Drawing for the job (mm, zero at the part's lowest x, y, z). A direction names the side the tool comes from. Give positions to 0.01 mm unless a question says otherwise; leave off trailing zeros. Write each loop counter-clockwise with the first axis right and the second up, starting at its lowest first coordinate (ties: lowest second). Pieces come first, ordered by that corner, then holes. Notation, with made-up numbers: (63.5, 9.5) - (81.5, 9.5) arc R21 cw to (81.5, 23.5) - close; hole circle Ø9 at (19, 15.25). An arc over 180 degrees is marked (long way). Write item = value, one per line. Start each with the question number.
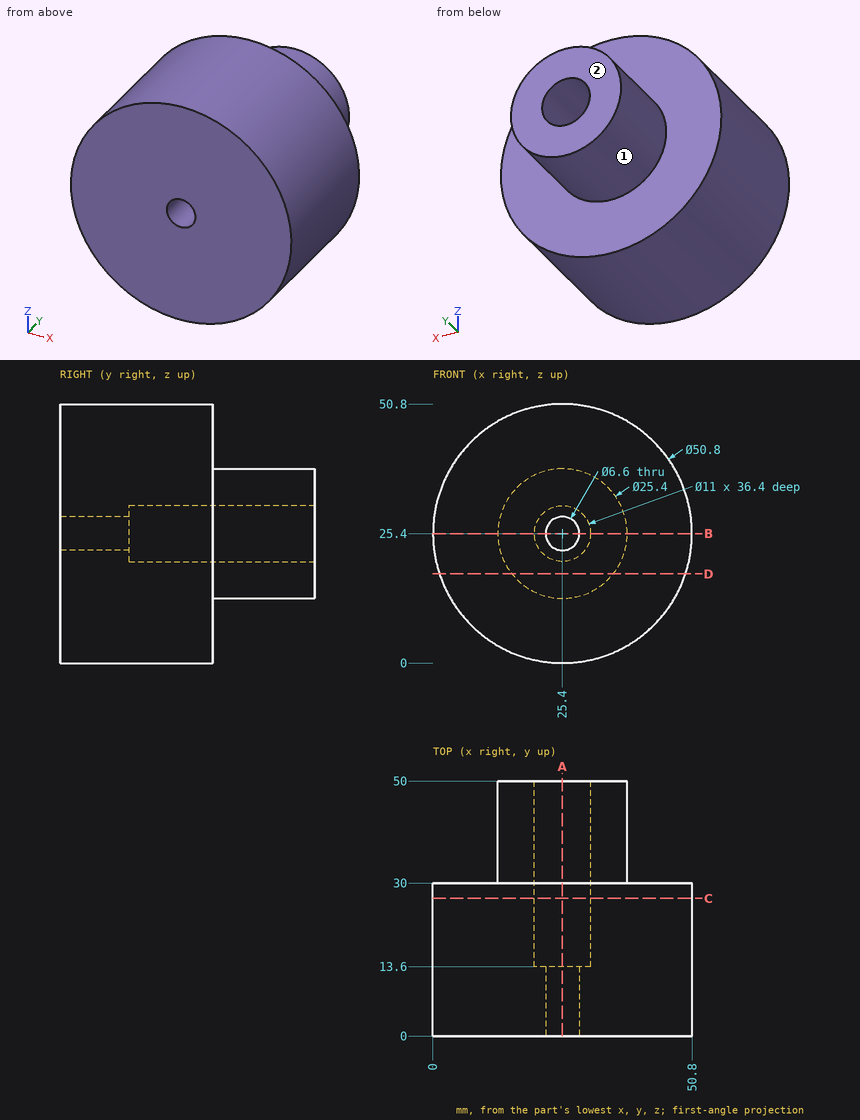
1. Pin check, flat tips, straight feed: pin 1 Ø5 at (x, y) = (11.5, 12.5) entering from -Z; pin 2 Ø1 at (y, z) = (37.5, 33) entering from +X; pin 3 Ø2 at (x, z) = (25.5, 7) entering from +Y. Stop position of each tip, or through.
2. Wall check: line 1 along X through (y, z) = (26, 25.4); line 2 along Y through (x, z) = (18, 14); line 3 along Z through (x, y) = (25.4, 34.5). Give the ranges that are in metal, low to high.
3. Cut at C-C (y = 27). Give the cut face in (x, z), then the cut area to 3 significant figures.
4. Cut at D-D (z = 17.5). Give the cut face in (x, y).
5. Cut at A-A (x = 25.4). Give the cut face in (y, z).
6. Cut at B-B (z = 25.4). Give the cut face in (x, y).
7. Tool access for the marked faces 1 and 2: list every direction of +Z, -Z, +X, -X, +Y, -Y with a clear straight run to the whole face (end or side of a thin tool).
Output:
q1.pin_1 = 2.7
q1.pin_2 = 35.93
q1.pin_3 = 30
q2.line_1 = 0 to 19.9, 30.9 to 50.8
q2.line_2 = 0 to 30
q2.line_3 = 12.7 to 19.9, 30.9 to 38.1
q3.outline = circle Ø50.8 at (25.4, 25.4); hole circle Ø11 at (25.4, 25.4)
q3.area = 1,930 mm2
q4.outline = (1.26, 0) - (49.54, 0) - (49.54, 30) - (35.34, 30) - (35.34, 50) - (15.46, 50) - (15.46, 30) - (1.26, 30) - close
q5.outline = (0, 0) - (30, 0) - (30, 12.7) - (50, 12.7) - (50, 19.9) - (13.6, 19.9) - (13.6, 22.1) - (0, 22.1) - close; (0, 28.7) - (13.6, 28.7) - (13.6, 30.9) - (50, 30.9) - (50, 38.1) - (30, 38.1) - (30, 50.8) - (0, 50.8) - close
q6.outline = (0, 0) - (22.1, 0) - (22.1, 13.6) - (19.9, 13.6) - (19.9, 50) - (12.7, 50) - (12.7, 30) - (0, 30) - close; (28.7, 0) - (50.8, 0) - (50.8, 30) - (38.1, 30) - (38.1, 50) - (30.9, 50) - (30.9, 13.6) - (28.7, 13.6) - close
q7.face_1 = +Y
q7.face_2 = +Z, -Z, +X, -X, +Y
